Verification items for this drawing (mm, ordinates from the low corner). A direction names the side the tool comes from. Give positions to 0.01 mm unless a question says otherwise; leave off trailing zeros. Order: outer loops, then holes, each group sorted by start corner. A loop starts at its lowest first (then second) coordinate and runs counter-clockwise, first axis right, second up.
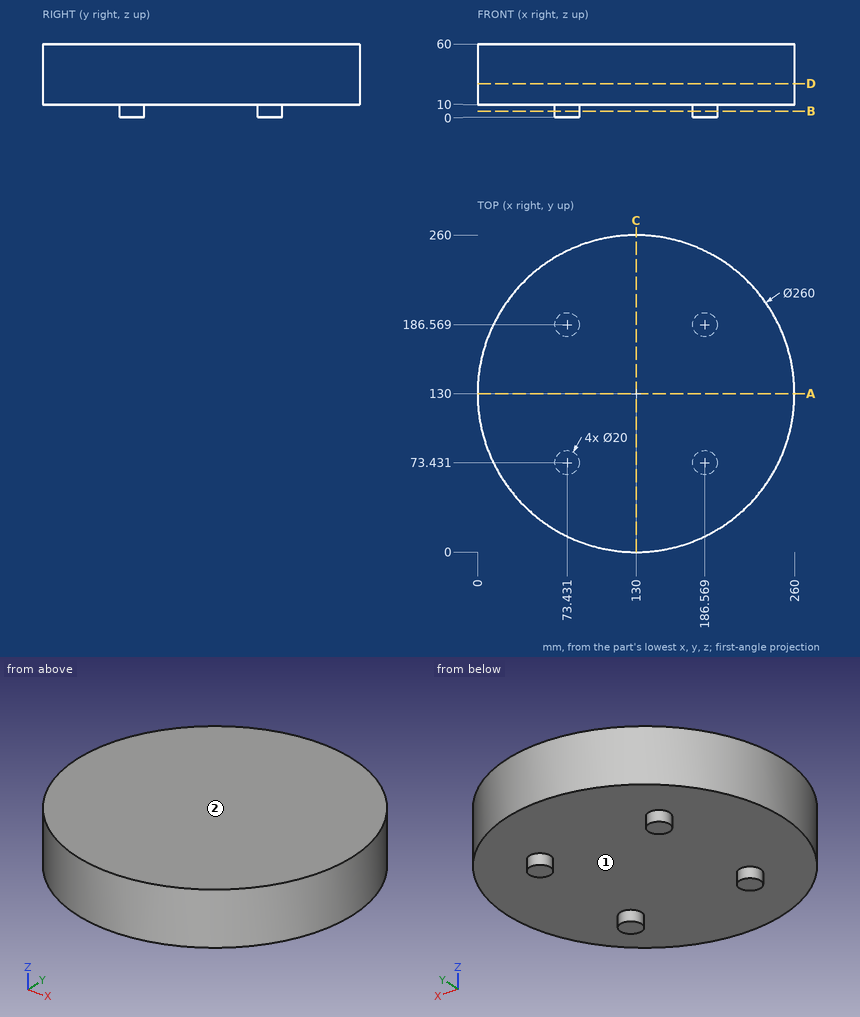
Q1. Access from +Z, -Z, +X, -X, +Y, -Y to the whole of each face (thin tool, end or side, straight path). Record for the marked faces 1 and 2.
Q2. Cross-section at B-B, the plane z = 5. Record the boundary of the cut face in (x, y), and give its area (3 significant figures).
Q3. Cross-section at D-D, the plane z = 27.5. Record the boundary of the cut face in (x, y).
Q4. Thickness scan on L1, parallel to Z at x = 207.5, y = 66.5; L2, parallel to Y at x = 100.5, z = 21.5; L3, parallel to Y at x = 219.5, z = 56 (1 decimal). Record the ranges inside material, lowest first.
Q5. Cross-section at A-A, the plane y = 130. Record the boundary of the cut face in (x, z), and give its area (3 significant figures).
Q6. Gauge pin test, flat ends, axial feed: P1, Ø8, axis at y = 199, z = 6.5, coming from the +X side (1 decimal); P2, Ø4, axis at x = 221, z = 51, coming from the +Y side; P3, Ø8, axis at y = 87, z = 48, coming from the +X side. Record the tip position at first contact, or that the pin passes through.
Answers follow:
1. face 1: -Z
1. face 2: +Z, +X, -X, +Y, -Y
2. outline: circle Ø20 at (73.43, 73.43); circle Ø20 at (73.43, 186.57); circle Ø20 at (186.57, 73.43); circle Ø20 at (186.57, 186.57)
2. area: 1,260 mm2
3. outline: circle Ø260 at (130, 130)
4. L1: z = 10 to 60
4. L2: y = 3.39 to 256.61
4. L3: y = 35.7 to 224.3
5. outline: (0, 10) - (260, 10) - (260, 60) - (0, 60) - close
5. area: 13,000 mm2
6. P1: stops at x = 241.4
6. P2: stops at y = 224.76
6. P3: stops at x = 254.01
